from build123d import *

# Parameters (mm, degrees)
SKETCH2_R           = 2.5527
BOSS_EXTRUDE1_DEPTH = 3.175


with BuildPart() as part:
    # Sketch2 → Boss-Extrude1 (new body)
    with BuildSketch(Plane(origin=(0, 0, 0), x_dir=(1, 0, 0), z_dir=(0, 1, 0))):
        with BuildLine():
            Line((-381, -147.6375), (-381, 147.6375))
            Line((-381, 147.6375), (-355.6, 147.6375))
            Line((-355.6, 147.6375), (-324.621785889, 178.615714111))
            ThreePointArc((-324.621785889, 178.615714111), (-313.457624236, 187.053879686), (-300.414699048, 192.125688655))
            ThreePointArc((-300.414699048, 192.125688655), (-271.668783425, 208.168783425), (-255.625688655, 236.914699048))
            ThreePointArc((-255.625688655, 236.914699048), (-250.553879686, 249.957624236), (-242.115714111, 261.121785889))
            Line((-242.115714111, 261.121785889), (-211.1375, 292.1))
            Line((-211.1375, 292.1), (-211.1375, 317.5))
            Line((-211.1375, 317.5), (211.1375, 317.5))
            Line((211.1375, 317.5), (211.1375, 292.1))
            Line((211.1375, 292.1), (242.115714111, 261.121785889))
            ThreePointArc((242.115714111, 261.121785889), (250.553879686, 249.957624236), (255.625688655, 236.914699048))
            ThreePointArc((255.625688655, 236.914699048), (271.668783425, 208.168783425), (300.414699048, 192.125688655))
            ThreePointArc((300.414699048, 192.125688655), (313.457624236, 187.053879686), (324.621785889, 178.615714111))
            Line((324.621785889, 178.615714111), (355.6, 147.6375))
            Line((355.6, 147.6375), (381, 147.6375))
            Line((381, 147.6375), (381, -147.6375))
            Line((381, -147.6375), (355.6, -147.6375))
            Line((355.6, -147.6375), (324.621785889, -178.615714111))
            ThreePointArc((324.621785889, -178.615714111), (313.457624236, -187.053879686), (300.414699048, -192.125688655))
            ThreePointArc((300.414699048, -192.125688655), (271.668783425, -208.168783425), (255.625688655, -236.914699048))
            ThreePointArc((255.625688655, -236.914699048), (250.553879686, -249.957624236), (242.115714111, -261.121785889))
            Line((242.115714111, -261.121785889), (211.1375, -292.1))
            Line((211.1375, -292.1), (211.1375, -317.5))
            Line((211.1375, -317.5), (-101.6, -317.5))
            Line((-101.6, -317.5), (-211.1375, -317.5))
            Line((-211.1375, -317.5), (-211.1375, -292.1))
            Line((-211.1375, -292.1), (-242.115714111, -261.121785889))
            ThreePointArc((-242.115714111, -261.121785889), (-250.553879686, -249.957624236), (-255.625688655, -236.914699048))
            ThreePointArc((-255.625688655, -236.914699048), (-271.668783425, -208.168783425), (-300.414699048, -192.125688655))
            ThreePointArc((-300.414699048, -192.125688655), (-313.457624236, -187.053879686), (-324.621785889, -178.615714111))
            Line((-324.621785889, -178.615714111), (-355.6, -147.6375))
            Line((-355.6, -147.6375), (-381, -147.6375))
        make_face()
        with Locations(Location((-190.5, 304.8, 0), (0, 0, 270))):
            Circle(SKETCH2_R, mode=Mode.SUBTRACT)
        with Locations(Location((-165.1, 304.8, 0), (0, 0, 270))):
            Circle(SKETCH2_R, mode=Mode.SUBTRACT)
        with Locations(Location((-139.7, 304.8, 0), (0, 0, 270))):
            Circle(SKETCH2_R, mode=Mode.SUBTRACT)
        with Locations(Location((-114.3, 304.8, 0), (0, 0, 270))):
            Circle(SKETCH2_R, mode=Mode.SUBTRACT)
        with Locations(Location((-88.9, 304.8, 0), (0, 0, 270))):
            Circle(SKETCH2_R, mode=Mode.SUBTRACT)
        with Locations(Location((-63.5, 304.8, 0), (0, 0, 270))):
            Circle(SKETCH2_R, mode=Mode.SUBTRACT)
        with Locations(Location((-38.1, 304.8, 0), (0, 0, 270))):
            Circle(SKETCH2_R, mode=Mode.SUBTRACT)
        with Locations(Location((-12.7, 304.8, 0), (0, 0, 270))):
            Circle(SKETCH2_R, mode=Mode.SUBTRACT)
        with Locations(Location((12.7, 304.8, 0), (0, 0, 270))):
            Circle(SKETCH2_R, mode=Mode.SUBTRACT)
        with Locations(Location((38.1, 304.8, 0), (0, 0, 270))):
            Circle(SKETCH2_R, mode=Mode.SUBTRACT)
        with Locations(Location((63.5, 304.8, 0), (0, 0, 270))):
            Circle(SKETCH2_R, mode=Mode.SUBTRACT)
        with Locations(Location((88.9, 304.8, 0), (0, 0, 270))):
            Circle(SKETCH2_R, mode=Mode.SUBTRACT)
        with Locations(Location((114.3, 304.8, 0), (0, 0, 270))):
            Circle(SKETCH2_R, mode=Mode.SUBTRACT)
        with Locations(Location((139.7, 304.8, 0), (0, 0, 270))):
            Circle(SKETCH2_R, mode=Mode.SUBTRACT)
        with Locations(Location((368.3, 127, 0), (0, 0, 270))):
            Circle(SKETCH2_R, mode=Mode.SUBTRACT)
        with Locations(Location((368.3, 101.6, 0), (0, 0, 270))):
            Circle(SKETCH2_R, mode=Mode.SUBTRACT)
        with Locations(Location((368.3, 76.2, 0), (0, 0, 270))):
            Circle(SKETCH2_R, mode=Mode.SUBTRACT)
        with Locations(Location((368.3, 50.8, 0), (0, 0, 270))):
            Circle(SKETCH2_R, mode=Mode.SUBTRACT)
        with Locations(Location((368.3, 25.4, 0), (0, 0, 270))):
            Circle(SKETCH2_R, mode=Mode.SUBTRACT)
        with Locations(Location((368.3, 0, 0), (0, 0, 270))):
            Circle(SKETCH2_R, mode=Mode.SUBTRACT)
        with Locations(Location((368.3, -25.4, 0), (0, 0, 270))):
            Circle(SKETCH2_R, mode=Mode.SUBTRACT)
        with Locations(Location((368.3, -50.8, 0), (0, 0, 270))):
            Circle(SKETCH2_R, mode=Mode.SUBTRACT)
        with Locations(Location((368.3, -76.2, 0), (0, 0, 270))):
            Circle(SKETCH2_R, mode=Mode.SUBTRACT)
        with Locations(Location((139.7, -304.8, 0), (0, 0, 90))):
            Circle(SKETCH2_R, mode=Mode.SUBTRACT)
        with Locations(Location((114.3, -304.8, 0), (0, 0, 90))):
            Circle(SKETCH2_R, mode=Mode.SUBTRACT)
        with Locations(Location((-114.3, -304.8, 0), (0, 0, 90))):
            Circle(SKETCH2_R, mode=Mode.SUBTRACT)
        with Locations(Location((-139.7, -304.8, 0), (0, 0, 90))):
            Circle(SKETCH2_R, mode=Mode.SUBTRACT)
        with Locations(Location((-165.1, -304.8, 0), (0, 0, 90))):
            Circle(SKETCH2_R, mode=Mode.SUBTRACT)
        with Locations(Location((-190.5, -304.8, 0), (0, 0, 90))):
            Circle(SKETCH2_R, mode=Mode.SUBTRACT)
        with Locations(Location((-368.3, -76.2, 0), (0, 0, 90))):
            Circle(SKETCH2_R, mode=Mode.SUBTRACT)
        with Locations(Location((-368.3, -50.8, 0), (0, 0, 90))):
            Circle(SKETCH2_R, mode=Mode.SUBTRACT)
        with Locations(Location((-368.3, -25.4, 0), (0, 0, 90))):
            Circle(SKETCH2_R, mode=Mode.SUBTRACT)
        with Locations(Location((-368.3, 0, 0), (0, 0, 90))):
            Circle(SKETCH2_R, mode=Mode.SUBTRACT)
        with Locations(Location((-368.3, 25.4, 0), (0, 0, 90))):
            Circle(SKETCH2_R, mode=Mode.SUBTRACT)
        with Locations(Location((-368.3, 50.8, 0), (0, 0, 90))):
            Circle(SKETCH2_R, mode=Mode.SUBTRACT)
        with Locations(Location((-368.3, 76.2, 0), (0, 0, 90))):
            Circle(SKETCH2_R, mode=Mode.SUBTRACT)
        with Locations(Location((-368.3, 101.6, 0), (0, 0, 90))):
            Circle(SKETCH2_R, mode=Mode.SUBTRACT)
        with Locations(Location((-368.3, 127, 0), (0, 0, 90))):
            Circle(SKETCH2_R, mode=Mode.SUBTRACT)
        with Locations(Location((-114.3, -279.4, 0), (0, 0, 270))):
            Circle(SKETCH2_R, mode=Mode.SUBTRACT)
        with Locations(Location((-114.3, -254, 0), (0, 0, 270))):
            Circle(SKETCH2_R, mode=Mode.SUBTRACT)
        with Locations(Location((-114.3, -228.6, 0), (0, 0, 270))):
            Circle(SKETCH2_R, mode=Mode.SUBTRACT)
        with Locations(Location((-114.3, -203.2, 0), (0, 0, 270))):
            Circle(SKETCH2_R, mode=Mode.SUBTRACT)
        with Locations(Location((-114.3, -177.8, 0), (0, 0, 270))):
            Circle(SKETCH2_R, mode=Mode.SUBTRACT)
        with Locations(Location((-114.3, -152.4, 0), (0, 0, 270))):
            Circle(SKETCH2_R, mode=Mode.SUBTRACT)
        with Locations(Location((-114.3, -127, 0), (0, 0, 270))):
            Circle(SKETCH2_R, mode=Mode.SUBTRACT)
        with Locations(Location((-114.3, -101.6, 0), (0, 0, 270))):
            Circle(SKETCH2_R, mode=Mode.SUBTRACT)
        with Locations(Location((114.3, -279.4, 0), (0, 0, 90))):
            Circle(SKETCH2_R, mode=Mode.SUBTRACT)
        with Locations(Location((114.3, -254, 0), (0, 0, 90))):
            Circle(SKETCH2_R, mode=Mode.SUBTRACT)
        with Locations(Location((114.3, -228.6, 0), (0, 0, 90))):
            Circle(SKETCH2_R, mode=Mode.SUBTRACT)
        with Locations(Location((114.3, -203.2, 0), (0, 0, 90))):
            Circle(SKETCH2_R, mode=Mode.SUBTRACT)
        with Locations(Location((114.3, -177.8, 0), (0, 0, 90))):
            Circle(SKETCH2_R, mode=Mode.SUBTRACT)
        with Locations(Location((114.3, -152.4, 0), (0, 0, 90))):
            Circle(SKETCH2_R, mode=Mode.SUBTRACT)
        with Locations(Location((114.3, -127, 0), (0, 0, 90))):
            Circle(SKETCH2_R, mode=Mode.SUBTRACT)
        with Locations(Location((114.3, -101.6, 0), (0, 0, 90))):
            Circle(SKETCH2_R, mode=Mode.SUBTRACT)
        with Locations(Location((165.1, 304.8, 0), (0, 0, 270))):
            Circle(SKETCH2_R, mode=Mode.SUBTRACT)
        with Locations(Location((190.5, 304.8, 0), (0, 0, 270))):
            Circle(SKETCH2_R, mode=Mode.SUBTRACT)
        with Locations(Location((368.3, -101.6, 0), (0, 0, 270))):
            Circle(SKETCH2_R, mode=Mode.SUBTRACT)
        with Locations(Location((368.3, -127, 0), (0, 0, 270))):
            Circle(SKETCH2_R, mode=Mode.SUBTRACT)
        with Locations(Location((165.1, -304.8, 0), (0, 0, 90))):
            Circle(SKETCH2_R, mode=Mode.SUBTRACT)
        with Locations(Location((190.5, -304.8, 0), (0, 0, 90))):
            Circle(SKETCH2_R, mode=Mode.SUBTRACT)
        with Locations(Location((-368.3, -101.6, 0), (0, 0, 90))):
            Circle(SKETCH2_R, mode=Mode.SUBTRACT)
        with Locations(Location((-368.3, -127, 0), (0, 0, 90))):
            Circle(SKETCH2_R, mode=Mode.SUBTRACT)
        with Locations(Location((-88.9, -304.8, 0), (0, 0, 90))):
            Circle(SKETCH2_R, mode=Mode.SUBTRACT)
        with Locations(Location((-63.5, -304.8, 0), (0, 0, 90))):
            Circle(SKETCH2_R, mode=Mode.SUBTRACT)
        with Locations(Location((-38.1, -304.8, 0), (0, 0, 90))):
            Circle(SKETCH2_R, mode=Mode.SUBTRACT)
        with Locations(Location((-12.7, -304.8, 0), (0, 0, 90))):
            Circle(SKETCH2_R, mode=Mode.SUBTRACT)
        with Locations(Location((12.7, -304.8, 0), (0, 0, 90))):
            Circle(SKETCH2_R, mode=Mode.SUBTRACT)
        with Locations(Location((38.1, -304.8, 0), (0, 0, 90))):
            Circle(SKETCH2_R, mode=Mode.SUBTRACT)
        with Locations(Location((63.5, -304.8, 0), (0, 0, 90))):
            Circle(SKETCH2_R, mode=Mode.SUBTRACT)
        with Locations(Location((88.9, -304.8, 0), (0, 0, 90))):
            Circle(SKETCH2_R, mode=Mode.SUBTRACT)
    extrude(amount=BOSS_EXTRUDE1_DEPTH)


solid = part.part
Could you check a few things on this model? Use its own coordinates, in mm. Coordinates: 2 decimals unless noted, no trailing zeros. Loops run counter-clockwise (first coordinate to the right, second up) from the corner with the lowest first, then second, coordinate; pieces in that order, holes last.
1. Imagine slicing it at A-A (y = 2.6). Give the number of separate pieces and of enclosed holes in the cut face, and give its area (3 significant figures).
2. For P1, Ø8, axis at x = -63.5, z = -304.8, coming from the +Y side (3 decimals); P2, Ø3, axis at x = 63.5, z = -304.8, coming from the +Y side; P3, Ø1.6, axis at x = 364.5, y = 1.5, coming from the +Z side, each with a flat end and sliding along its axis, tell me the tip position at first contact or that it passes through.
3. Imagine slicing it at C-C (x = -265.5). Please give me the cut outline in (y, z) (3 decimals), and give its area (3 significant figures).
4. We'd pull the mould along X, two halves only. Please class faces 1 (the face through (-226.41, 1.57, 276.83)), 2 (the face through (340.33, 1.57, 162.91)), 3 (the face through (5, 0, -4)): released by +X, released by -X, zero draft, split by the parting line, or undercut.
5. Imagine slicing it at B-B (z = -277.5). Please give me the cut outline in (x, y) (1 decimal), and give its area (3 significant figures).
6. I need wall thicknesses on L1, parallel to X at y = 1.1, z = 25.4; L2, parallel to Z at x = -165.5, y = 2; L3, parallel to Z at x = 190.5, y = 0.95. Which ranges of each line are inside material? Lowest first, please.
Computed values:
1. separate pieces: 1
1. enclosed holes: 70
1. area: 405,000 mm2
2. P1: stops at y = 3.175
2. P2: passes through
2. P3: stops at z = 147.64
3. outline: (0, -215.396) - (3.175, -215.396) - (3.175, 215.396) - (0, 215.396) - close
3. area: 1,370 mm2
4. face 1: released by -X
4. face 2: released by +X
4. face 3: zero draft
5. outline: (-225.7, 0) - (225.7, 0) - (225.7, 3.2) - (-225.7, 3.2) - close
5. area: 1,430 mm2
6. L1: x = -381 to -370.85, -365.75 to 365.75, 370.85 to 381
6. L2: z = -317.5 to -307.32, -302.28 to 302.28, 307.32 to 317.5
6. L3: z = -317.5 to -307.35, -302.25 to 302.25, 307.35 to 317.5
